Could you check a few things on this drawing? It's one solid part, dimensions in mm from its lowest x, y, z. A direction names the side the tool comes from. Round coordinates to 2 decimals unless told otherwise and drop trailing zeros. Order: outer loops, then holes, each group sorted by start corner. A loop starts at its lowest first (then second) coordinate and runs counter-clockwise, first axis right, second up. Notation, with made-up numbers: (72, 28) - (78, 28) arc R38 cw to (78, 67) - close; hole circle Ø8 at (23, -6). An arc over 180 degrees is marked (long way). Use one line per item in the form item = value.
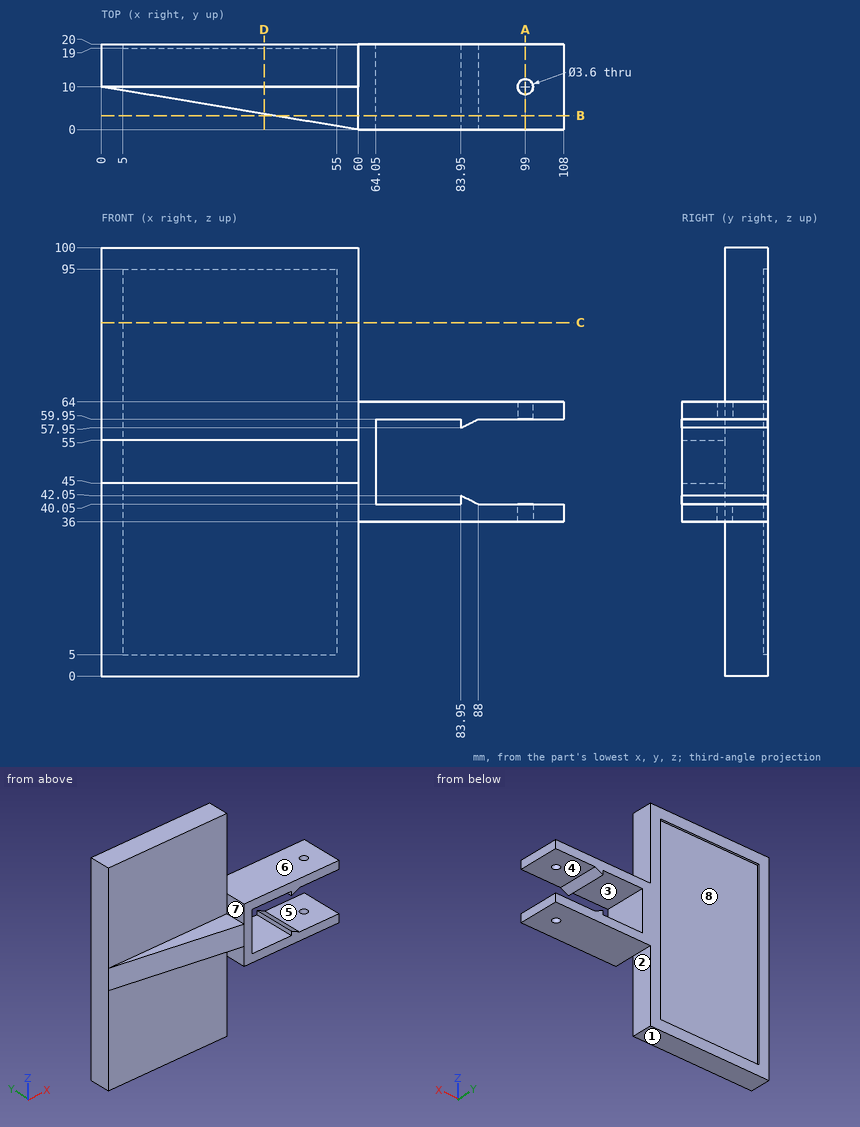
Item 1: If we mould it in two halves opening along Z, with no side actions, what happens to the marked faces 1, 2, 3 and 4? For each: released by +Z, released by -Z, zero draft, split by the parting line, or undercut.
Found:
face_1 = released by -Z
face_2 = zero draft
face_3 = undercut
face_4 = undercut
Item 2: For the marked faces 5, 6, 7 and 8, which set-ups out of +Z, -Z, +X, -X, +Y, -Y let a thin tool reach every point of the face, with its end or its side?
Found:
face_5 = +X, +Y, -Y
face_6 = +Z, +X, +Y, -Y
face_7 = +Z, -X, -Y
face_8 = +Y
Item 3: Imagine slicing it at D-D on x = 38. Please give me the cut outline in (y, z), plus the area to 3 significant figures.
Found:
outline = (3.67, 45) - (10, 45) - (10, 0) - (20, 0) - (20, 5) - (19, 5) - (19, 95) - (20, 95) - (20, 100) - (10, 100) - (10, 55) - (3.67, 55) - close
area = 973 mm2
Item 4: Imagine slicing it at A-A on x = 99. Please give me the cut outline in (y, z).
Found:
outline = (0, 36) - (8.2, 36) - (8.2, 40.05) - (0, 40.05) - close; (0, 59.95) - (8.2, 59.95) - (8.2, 64) - (0, 64) - close; (11.8, 36) - (20, 36) - (20, 40.05) - (11.8, 40.05) - close; (11.8, 59.95) - (20, 59.95) - (20, 64) - (11.8, 64) - close
Item 5: Will these pins go through, and if not, where does the flat tip stop? P1, Ø1, axis at y = 13.5, z = 41.5, coming from the -X side; P2, Ø4, axis at y = 4, z = 51.5, coming from the +X side; P3, Ø8, axis at y = 17, z = 12, coming from the +X side; P4, Ø3, axis at x = 99, y = 10, coming from the -Z side.
Found:
P1 = 0
P2 = 64.05
P3 = 60
P4 = through
Item 6: Imagine slicing it at C-C on z = 82.5. Please give me the cut outline in (x, y).
Found:
outline = (0, 10) - (60, 10) - (60, 20) - (55, 20) - (55, 19) - (5, 19) - (5, 20) - (0, 20) - close
Item 7: Imagine slicing it at B-B on y = 3.25. Please give me the cut outline in (x, z).
Found:
outline = (40.5, 45) - (60, 45) - (60, 36) - (108, 36) - (108, 40.05) - (88, 40.05) - (83.95, 42.05) - (83.95, 40.05) - (64.05, 40.05) - (64.05, 59.95) - (83.95, 59.95) - (83.95, 57.95) - (88, 59.95) - (108, 59.95) - (108, 64) - (60, 64) - (60, 55) - (40.5, 55) - close
Item 8: I need wall thicknesses on L1, parallel to Z at x = 82.5, y = 19; L2, parallel to Y at x = 99, z = 37.75; L3, parallel to X at y = 19.25, z = 27.5. Which ranges of each line are inside material? Lowest first, please.
Found:
L1 = 36 to 40.05, 59.95 to 64
L2 = 0 to 8.2, 11.8 to 20
L3 = 0 to 5, 55 to 60
